```python
from build123d import *

# Parameters (mm, degrees)
CYLINDER_R     = 20
CYLINDER_DEPTH = 200


with BuildPart() as cylinder:
    # Cylinder → Cylinder (new body)
    with BuildSketch(Plane.XY.offset(-100)):
        Circle(CYLINDER_R)
    extrude(amount=CYLINDER_DEPTH)


with BuildPart() as sphere001:
    # Sphere001 → Sphere001 (revolve)
    with BuildSketch(Plane(origin=(0, 0, -36.754386), x_dir=(1, 0, 0), z_dir=(0, -1, 0))):
        with BuildLine():
            ThreePointArc((0, -44.105263), (44.105263, 0), (0, 44.105263))
            Line((0, 44.105263), (0, -44.105263))
        make_face()
    revolve(axis=Axis((0, 0, -36.754386), (0, 0, 1)))


with BuildPart() as common001:
    # Sphere → Sphere (revolve)
    with BuildSketch(Plane(origin=(0, 0, 36.754386), x_dir=(1, 0, 0), z_dir=(0, -1, 0))):
        with BuildLine():
            ThreePointArc((0, -44.105263), (44.105263, 0), (0, 44.105263))
            Line((0, 44.105263), (0, -44.105263))
        make_face()
    revolve(axis=Axis((0, 0, 36.754386), (0, 0, 1)))

    # Common: intersect Sphere001
    add(sphere001.part, mode=Mode.INTERSECT)

    # Common001: intersect Cylinder
    add(cylinder.part, mode=Mode.INTERSECT)


with BuildPart() as common001_1:
    # Common001 placement: moved
    add(common001.part.moved(Location((0, 0, -50))))


solid = common001_1.part
```
For this review, take the finished solid that the model builds, in its own axes (mm). Round coordinates to 2 decimals unless told otherwise and drop trailing zeros. Loops run counter-clockwise (first coordinate to the right, second up) from the corner with the lowest first, then second, coordinate; pieces in that order, holes last.
Q1. Add section D-D on z = -54.75. Write out the cut boundary in (x, y), plus the area to 3 significant figures.
Result sheet:
outline: circle Ø29.84 at (0, 0)
area: 700 mm2
Q2. Add section A-A on x = 0. Write out the cut boundary in (y, z), plus the area to 3 significant figures.
Result sheet:
outline: (-20, -52.56) arc R44.11 ccw to (20, -52.56) - (20, -47.44) arc R44.11 ccw to (-20, -47.44) - close
area: 463 mm2
Q3. Add section C-C on z = -52. Write out the cut boundary in (x, y).
Result sheet:
outline: circle Ø40 at (0, 0)
Q4. To check wall thickness, follow line 1 along X through (y, z) = (-4, -53.25); line 2 along X through (y, z) = (10.5, -52.75); line 3 along Y through (x, z) = (-0.5, -48.75). State the ranges of each line that lie inside material, in increasing order.
Result sheet:
line 1: x = -18.14 to 18.14
line 2: x = -16.57 to 16.57
line 3: y = -19.99 to 19.99
Q5. Insertion check: pin 1 Ø4 at (y, z) = (-15.5, -49) entering from -X; pin 2 Ø5 at (x, y) = (-3.5, -14) entering from -Z; pin 3 Ø2 at (y, z) = (-2, -45) entering from -X. Each pin has a flat end and moves straight along its axis. Give the tip position at first contact, or say it passes through.
Result sheet:
pin 1: stops at x = -14.76
pin 2: stops at z = -55.71
pin 3: stops at x = -16.75
